from build123d import *

# Parameters (mm, degrees)
BOSS_EXTRUDE1_DEPTH = 5
CUT_EXTRUDE1_DEPTH  = 3


with BuildPart() as part:
    # Sketch1 → Boss-Extrude1 (new body)
    with BuildSketch(Plane(origin=(0, 0, 0), x_dir=(1, 0, 0), z_dir=(0, 1, 0))):
        Polygon((0, -55), (60, -55), (60, -33.5), (140, -33.5), (140, -24), (60, -24), (60, 0), (45, 0), (45, -40), (15, -40), (15, 0), (0, 0), align=None)
    extrude(amount=BOSS_EXTRUDE1_DEPTH)

    # Sketch4 → Cut-Extrude1 (cut)
    # profile 1 of 6: a face of its own
    with BuildSketch(Plane(origin=(0, 5, 0), x_dir=(1, 0, 0), z_dir=(0, 1, 0))):
        Polygon((12.435897436, -49), (10.58974359, -45), (10.979967949, -45), (11.571314103, -46.282051282), (13.384615385, -46.282051282), (13.992788462, -45), (14.384615385, -45), (12.487179487, -49), align=None)
        Polygon((12.465544872, -48.220352564), (13.189903846, -46.692307692), (11.760416667, -46.692307692), align=None, mode=Mode.SUBTRACT)
    # profile 2 of 6: a face of its own
    with BuildSketch(Plane(origin=(0, 5, 0), x_dir=(1, 0, 0), z_dir=(0, 1, 0))):
        Polygon((21.225641026, -45), (21.225641026, -49), (21.150320513, -49), (18.507692308, -45.851762821), (18.507692308, -49), (18.148717949, -49), (18.148717949, -45), (18.230448718, -45), (20.866666667, -48.141025641), (20.866666667, -45), align=None)
    # profile 3 of 6: a face of its own
    with BuildSketch(Plane(origin=(0, 5, 0), x_dir=(1, 0, 0), z_dir=(0, 1, 0))):
        Polygon((26.733333333, -49), (24.887179487, -45), (25.277403846, -45), (25.86875, -46.282051282), (27.682051282, -46.282051282), (28.290224359, -45), (28.682051282, -45), (26.784615385, -49), align=None)
        Polygon((26.762980769, -48.220352564), (27.487339744, -46.692307692), (26.057852564, -46.692307692), align=None, mode=Mode.SUBTRACT)
    # profile 4 of 6: a face of its own
    with BuildSketch(Plane(origin=(0, 5, 0), x_dir=(1, 0, 0), z_dir=(0, 1, 0))):
        Polygon((35.523076923, -45), (35.523076923, -49), (35.44775641, -49), (32.805128205, -45.851762821), (32.805128205, -49), (32.446153846, -49), (32.446153846, -45), (32.527884615, -45), (35.164102564, -48.141025641), (35.164102564, -45), align=None)
    # profile 5 of 6: a face of its own
    with BuildSketch(Plane(origin=(0, 5, 0), x_dir=(1, 0, 0), z_dir=(0, 1, 0))):
        Polygon((41.030769231, -49), (39.184615385, -45), (39.574839744, -45), (40.166185897, -46.282051282), (41.979487179, -46.282051282), (42.587660256, -45), (42.979487179, -45), (41.082051282, -49), align=None)
        Polygon((41.060416667, -48.220352564), (41.784775641, -46.692307692), (40.355288462, -46.692307692), align=None, mode=Mode.SUBTRACT)
    # profile 6 of 6: a face of its own
    with BuildSketch(Plane(origin=(0, 5, 0), x_dir=(1, 0, 0), z_dir=(0, 1, 0))):
        with BuildLine():
            Line((48.897435897, -49), (48.116987179, -49))
            add(Edge.make_bspline(
                [(48.116987179, -49), (48.078782602, -48.999802304), (48.004732622, -48.999419121), (47.897061448, -48.993338284), (47.7961773, -48.985254385), (47.702258451, -48.97169408), (47.614693787, -48.957633832), (47.534372273, -48.936996754), (47.460621116, -48.91420235), (47.372061071, -48.879130066), (47.271577566, -48.824662366), (47.163576599, -48.743881592), (47.06969557, -48.647031967), (46.989868866, -48.536664179), (46.925806239, -48.415247106), (46.880046085, -48.285393075), (46.85064802, -48.149286724), (46.847662619, -48.055973237), (46.846153846, -48.008814103)],
                knots=[0, 0, 0, 0, 1.00128172, 1.940733171, 2.826250472, 3.653024905, 4.427672124, 5.149348099, 5.824709082, 6.450061444, 7.643590664, 8.808605388, 9.972104426, 11.165284501, 12.367876273, 13.557044126, 14.765369432, 16, 16, 16, 16], degree=3))
            add(Edge.make_bspline(
                [(46.846153846, -48.008814103), (46.847386233, -47.964634112), (46.84980799, -47.877816264), (46.873466598, -47.751260803), (46.909178693, -47.630411683), (46.960713415, -47.516433521), (47.026424516, -47.410327841), (47.106371945, -47.313904536), (47.201167683, -47.22905671), (47.272340847, -47.181837688), (47.30849359, -47.157852564)],
                knots=[0, 0, 0, 0, 1.044356178, 2.052258378, 3.035953355, 4.020338374, 5.002448483, 5.980768927, 6.974322109, 8, 8, 8, 8], degree=3))
            add(Edge.make_bspline(
                [(47.30849359, -47.157852564), (47.263049876, -47.140414673), (47.176104795, -47.107051668), (47.056302302, -47.047837808), (46.953049503, -46.983927334), (46.86501575, -46.9148518), (46.791249685, -46.838355693), (46.725535913, -46.756453592), (46.669766654, -46.666293122), (46.622183034, -46.56982802), (46.584489246, -46.467569127), (46.558324516, -46.360281463), (46.54173076, -46.249180208), (46.539560824, -46.173670002), (46.538461538, -46.135416667)],
                knots=[0, 0, 0, 0, 1.272200328, 2.434034374, 3.488177493, 4.442517805, 5.351202203, 6.260825393, 7.183200622, 8.11705787, 9.069326169, 10.026320267, 11.000137371, 12, 12, 12, 12], degree=3))
            add(Edge.make_bspline(
                [(46.538461538, -46.135416667), (46.539578041, -46.096368878), (46.541774791, -46.019541259), (46.557978943, -45.90667732), (46.585423547, -45.798823648), (46.623198448, -45.695262323), (46.672439932, -45.596599873), (46.731928763, -45.502060921), (46.803327906, -45.413046548), (46.883730364, -45.328265046), (46.973436376, -45.250736025), (47.072285382, -45.184110133), (47.177743985, -45.126562612), (47.291256316, -45.080297632), (47.412016926, -45.044080616), (47.540054106, -45.019040231), (47.675295151, -45.002100252), (47.768107642, -45.000711963), (47.815705128, -45)],
                knots=[0, 0, 0, 0, 0.978522333, 1.925270105, 2.85076145, 3.763600118, 4.682725947, 5.609499657, 6.557784645, 7.537954401, 8.534920712, 9.522742111, 10.520247711, 11.5409147, 12.58930695, 13.675078472, 14.807699069, 16, 16, 16, 16], degree=3))
            Line((47.815705128, -45), (48.897435897, -45))
            Line((48.897435897, -45), (48.897435897, -49))
        make_face()
        with BuildLine():
            Line((48.538461538, -48.58974359), (48.538461538, -47.307692308))
            Line((48.538461538, -47.307692308), (48.297275641, -47.307692308))
            add(Edge.make_bspline(
                [(48.297275641, -47.307692308), (48.262019557, -47.308145559), (48.193897619, -47.309021333), (48.094984144, -47.311609081), (48.003398634, -47.318537578), (47.918825519, -47.32586562), (47.841831582, -47.337149257), (47.772159281, -47.350957405), (47.709182048, -47.365432661), (47.636590639, -47.390121207), (47.554259533, -47.426226355), (47.46710675, -47.483630694), (47.388665327, -47.550092509), (47.323955681, -47.628926607), (47.270082552, -47.714060303), (47.233811866, -47.806128442), (47.208522595, -47.901958331), (47.206271259, -47.968047579), (47.205128205, -48.001602564)],
                knots=[0, 0, 0, 0, 1.156584208, 2.234756387, 3.244705828, 4.168772894, 5.018724976, 5.795346628, 6.498686023, 7.135894168, 8.308330183, 9.43588092, 10.547699294, 11.667188675, 12.76860303, 13.837480448, 14.902040606, 16, 16, 16, 16], degree=3))
            add(Edge.make_bspline(
                [(47.205128205, -48.001602564), (47.205685691, -48.023816697), (47.20677926, -48.067392143), (47.217088766, -48.130879067), (47.231315761, -48.191293527), (47.25477962, -48.247006859), (47.282578229, -48.299975385), (47.318209405, -48.34852593), (47.359295429, -48.393973734), (47.407196584, -48.435100612), (47.461717059, -48.472297499), (47.524583935, -48.503262131), (47.594088014, -48.530780023), (47.671678673, -48.551639229), (47.755810377, -48.569748341), (47.847766678, -48.581167846), (47.946993383, -48.588503916), (48.015743783, -48.589321148), (48.051282051, -48.58974359)],
                knots=[0, 0, 0, 0, 0.911412742, 1.787835618, 2.63643285, 3.453173233, 4.262886967, 5.08783453, 5.918594724, 6.773969545, 7.67442701, 8.62112486, 9.645634318, 10.739428598, 11.916091468, 13.177237585, 14.540865421, 16, 16, 16, 16], degree=3))
            Line((48.051282051, -48.58974359), (48.538461538, -48.58974359))
        make_face(mode=Mode.SUBTRACT)
        with BuildLine():
            Line((48.538461538, -46.897435897), (48.538461538, -45.41025641))
            Line((48.538461538, -45.41025641), (48.02724359, -45.41025641))
            add(Edge.make_bspline(
                [(48.02724359, -45.41025641), (47.99065419, -45.41073715), (47.920132945, -45.411663713), (47.818234921, -45.41386232), (47.724292741, -45.422019142), (47.63752424, -45.429839399), (47.558330886, -45.442615415), (47.485942388, -45.454987006), (47.422012134, -45.473192413), (47.347210045, -45.498243376), (47.26354466, -45.538278135), (47.172178111, -45.597152678), (47.091703188, -45.66886621), (47.023425854, -45.751440271), (46.966656245, -45.84029687), (46.927382886, -45.935610894), (46.901935986, -46.034198698), (46.898938947, -46.101609423), (46.897435897, -46.135416667)],
                knots=[0, 0, 0, 0, 1.16016216, 2.236059617, 3.229676189, 4.14889023, 4.996733752, 5.772278665, 6.474820656, 7.101410824, 8.271817372, 9.403828207, 10.537358096, 11.673541442, 12.791884111, 13.865947414, 14.929748409, 16, 16, 16, 16], degree=3))
            add(Edge.make_bspline(
                [(46.897435897, -46.135416667), (46.897742716, -46.156555083), (46.898351404, -46.198490951), (46.907919371, -46.260062814), (46.921197263, -46.320001273), (46.940765146, -46.377492166), (46.964436964, -46.433525476), (46.995666123, -46.486277982), (47.030892383, -46.537995275), (47.085452532, -46.604147419), (47.165892911, -46.679445819), (47.280241748, -46.752246439), (47.409533392, -46.811908817), (47.503528097, -46.837131085), (47.552083333, -46.850160256)],
                knots=[0, 0, 0, 0, 0.723354195, 1.435040621, 2.129761981, 2.824182007, 3.512608497, 4.209435533, 4.920062464, 5.654614313, 7.143585817, 8.671381114, 10.280521501, 12, 12, 12, 12], degree=3))
            add(Edge.make_bspline(
                [(47.552083333, -46.850160256), (47.571545139, -46.854109189), (47.613742348, -46.86267129), (47.682551361, -46.871703561), (47.76137005, -46.879805803), (47.849861531, -46.88564168), (47.948377746, -46.891906393), (48.056887045, -46.894256042), (48.175466139, -46.897123913), (48.257743237, -46.897329242), (48.300480769, -46.897435897)],
                knots=[0, 0, 0, 0, 0.634452549, 1.375623993, 2.216454381, 3.166361212, 4.209414599, 5.370755378, 6.634280627, 8, 8, 8, 8], degree=3))
            Line((48.300480769, -46.897435897), (48.538461538, -46.897435897))
        make_face(mode=Mode.SUBTRACT)
    extrude(amount=-CUT_EXTRUDE1_DEPTH, mode=Mode.SUBTRACT)


solid = part.part
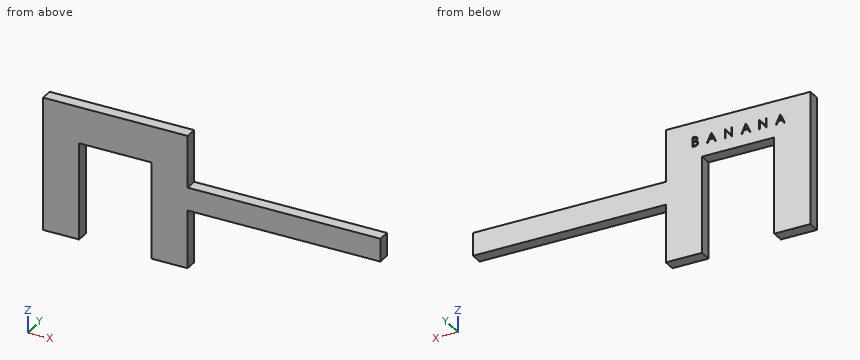
Geometry: final body of the model. Coordinates: model frame, mm. Give positions to 0.01 mm unless a question says otherwise; leave off trailing zeros. Loops run counter-clockwise (first coordinate to the right, second up) from the corner with the lowest first, then second, coordinate; pieces in that order, holes last. Notation, with made-up numbers: (41, 52) - (62, 52) arc R16 ccw to (62, 74) - close; hole circle Ø10 at (77.25, 48.5). An arc over 180 degrees is marked (long way). Answer as CSV lines item,"result". Start each with the question number.
1. Section C-C, the plane z = 41.5. Return loops of the section in (x, y), plus the area to 3 significant figures.
2. Section B-B, the plane y = 0.9. Return loops of the section in (x, z), plus the area to 3 significant figures.
3. Ray query, L1, parallel to X at y = 0.25, z = 16.5; L2, parallel to Z at x = 28.5, y = 2.2; L3, parallel to Z at x = 108.5, y = 4.6. Return the intervals inside material, ascending.
4. Section D-D, the plane z = 20.5. Return loops of the section in (x, y).
5. Pin query (flat end, axial travel): P1, Ø2, axis at x = 125.5, y = 4.5, coming from the +Z side; P2, Ø0.7, axis at y = 4, z = 46.5, coming from the +X side. Return the tip coordinate at first contact, or that it passes through.
6. Section A-A, the plane z = 31. Return loops of the section in (x, y).
Answers:
1,outline,"(0, 0) - (60, 0) - (60, 5) - (0, 5) - close"
1,area,"300 mm2"
2,outline,"(0, 0) - (15, 0) - (15, 40) - (45, 40) - (45, 0) - (60, 0) - (60, 24) - (140, 24) - (140, 33.5) - (60, 33.5) - (60, 55) - (0, 55) - close"
2,area,"2,860 mm2"
3,L1,"x = 0 to 15, 45 to 60"
3,L2,"z = 40 to 45, 45.38 to 55"
3,L3,"z = 24 to 33.5"
4,outline,"(0, 0) - (15, 0) - (15, 5) - (0, 5) - close; (45, 0) - (60, 0) - (60, 5) - (45, 5) - close"
5,P1,"stops at z = 33.5"
5,P2,"stops at x = 60"
6,outline,"(0, 0) - (15, 0) - (15, 5) - (0, 5) - close; (45, 0) - (140, 0) - (140, 5) - (45, 5) - close"
